Part model, mm, in its own coordinate system. Face numbers are marked on the shaded views. Give positions to 0.01 mm unless a question says otherwise; leave off trailing zeros. Loops run counter-clockwise (first coordinate to the right, second up) from the corner with the lowest first, then second, coordinate; pieces in that order, holes last. Notation, with made-up numbers: (27.25, 24) -> (53.25, 24) arc R17 cw to (53.25, 40) -> close; hole circle Ø2 at (25, -19). An arc over 180 degrees is marked (long way). One line per question, with ' | ' between items.
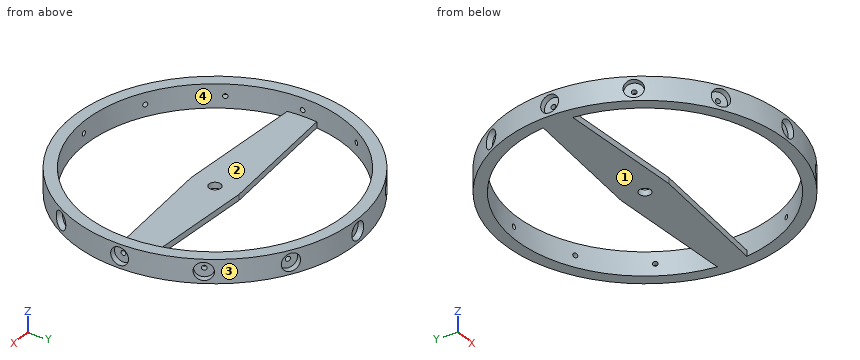
```python
from build123d import *

# Parameters (mm, degrees)
CROQUIS1_R              = 6
CROQUIS1_R_2            = 5.5
SALIENTE_EXTRUIR1_DEPTH = 1
SALIENTE_EXTRUIR2_DEPTH = 0.25
CROQUIS8_R              = 0.1
CORTAR_EXTRUIR4_DEPTH   = 1
CROQUIS9_R              = 0.375
CORTAR_EXTRUIR5_DEPTH   = 0.25
MATRIZC7_COUNT          = 12
CROQUIS10_R             = 0.25
CORTAR_EXTRUIR6_DEPTH   = 10


with BuildPart() as part:
    # Croquis1 → Saliente-Extruir1 (new body)
    with BuildSketch(Plane.XY):
        Circle(CROQUIS1_R)
        Circle(CROQUIS1_R_2, mode=Mode.SUBTRACT)
    extrude(amount=SALIENTE_EXTRUIR1_DEPTH)

    # Croquis5 → Saliente-Extruir2 (add)
    with BuildSketch(Plane.XY):
        with BuildLine():
            Line((0, 1), (0, -1))
            Line((0, -1), (5.465187795, -0.617836841))
            ThreePointArc((5.465187795, -0.617836841), (5.5, 0), (5.465187795, 0.617836841))
            Line((5.465187795, 0.617836841), (0, 1))
        make_face()
    saliente_extruir2 = extrude(amount=SALIENTE_EXTRUIR2_DEPTH)

    # Simetría1: Saliente-Extruir2 across Right Plane
    add(saliente_extruir2.mirror(Plane(origin=(0, 0, 0), x_dir=(0, 0, -1), z_dir=(1, 0, 0))))

    # Croquis8 → Cortar-Extruir4 (cut)
    with BuildSketch(Plane(origin=(0, 6, 0), x_dir=(-1, 0, 0), z_dir=(0, 1, 0))):
        with Locations((0, 0.5)):
            Circle(CROQUIS8_R)
    cortar_extruir4 = extrude(amount=-CORTAR_EXTRUIR4_DEPTH, mode=Mode.SUBTRACT)

    # Croquis9 → Cortar-Extruir5 (cut)
    with BuildSketch(Plane(origin=(0, 6, 0), x_dir=(-1, 0, 0), z_dir=(0, 1, 0))):
        with Locations((0, 0.5)):
            Circle(CROQUIS9_R)
    cortar_extruir5 = extrude(amount=-CORTAR_EXTRUIR5_DEPTH, mode=Mode.SUBTRACT)

    # MatrizC7: Cortar-Extruir4, Cortar-Extruir5 ×12 about axis
    matrizc7_axis = Axis((0, 0, 0), (0, 0, 1))
    for i in range(1, MATRIZC7_COUNT):
        add(cortar_extruir4.rotate(matrizc7_axis, i * 360 / MATRIZC7_COUNT), mode=Mode.SUBTRACT)
        add(cortar_extruir5.rotate(matrizc7_axis, i * 360 / MATRIZC7_COUNT), mode=Mode.SUBTRACT)

    # Croquis10 → Cortar-Extruir6 (cut)
    with BuildSketch(Plane(origin=(0, 0, 0), x_dir=(-1, 0, 0), z_dir=(0, 0, -1))):
        Circle(CROQUIS10_R)
    extrude(amount=-CORTAR_EXTRUIR6_DEPTH, mode=Mode.SUBTRACT)


solid = part.part
```
1) Pin check, flat tips, straight feed: P1, Ø0.6, axis at x = 0, z = 0.5, coming from the -Y side; P2, Ø4, axis at x = -3, y = 0, coming from the +Z side; P3, Ø0.6, axis at y = 0, z = 0.5, coming from the +X side. Stop position of each tip, or through.
Found:
P1: y = -5.75 | P2: z = 0.25 | P3: x = 5.75
2) Saw through at A-A (y = 4). Give the cut face in (x, z), and give its area (3 significant figures).
Found:
outline: (-4.47, 0) -> (-3.77, 0) -> (-3.77, 1) -> (-4.47, 1) -> close; (3.77, 0) -> (4.47, 0) -> (4.47, 1) -> (3.77, 1) -> close | area: 1.39 mm2
3) Saw through at D-D (y = -1.25). Give the cut face in (x, z), and give its area (3 significant figures).
Found:
outline: (-5.87, 0) -> (-5.36, 0) -> (-5.36, 1) -> (-5.87, 1) -> close; (5.36, 0) -> (5.87, 0) -> (5.87, 1) -> (5.36, 1) -> close | area: 1.02 mm2
4) Pull direction X, two halves, no side cores. Call the marked faces 1, 2, 3 and 4: pulls with the +X half, pulls with the -X half, needs draft (parallel to the pull), parting line crosses it, or undercut.
Found:
face 1: needs draft | face 2: undercut | face 3: parting line crosses it | face 4: undercut
5) Saw through at C-C (x = -4.25). Give the cut face in (y, z), and give its area (3 significant figures).
Found:
outline: (-4.24, 0) -> (-3.49, 0) -> (-3.49, 1) -> (-4.24, 1) -> close; (-0.7, 0) -> (0.7, 0) -> (0.7, 0.25) -> (-0.7, 0.25) -> close; (3.49, 0) -> (4.24, 0) -> (4.24, 1) -> (3.49, 1) -> close | area: 1.84 mm2
6) Drill centre lines: line 1 (Y direction, x = -2, z = 0.15); line 2 (Z direction, x = 0, y = -5.55); line 3 (Y direction, x = 1.75, z = 0.8). Where is each one in solid material? Low to high.
Found:
line 1: -5.66 to -5.12, -0.86 to 0.86, 5.12 to 5.66 | line 2: 0 to 0.4, 0.6 to 1 | line 3: -5.74 to -5.21, 5.21 to 5.74
7) Saw through at B-B (x = 3.75). Give the cut face in (y, z).
Found:
outline: (-4.68, 0) -> (-4.02, 0) -> (-4.02, 1) -> (-4.68, 1) -> close; (-0.74, 0) -> (0.74, 0) -> (0.74, 0.25) -> (-0.74, 0.25) -> close; (4.02, 0) -> (4.68, 0) -> (4.68, 1) -> (4.02, 1) -> close
